Autodesk Inventor part; units mm, degrees
ref_plane "Начальная плоскость" through (0, 0, 0) normal (0, 0, 1) x (1, 0, 0)
ref_plane "Конечная плоскость" through (0, 0, 1) normal (0, 0, 1) x (1, 0, 0)
ref_plane "YZ Plane" through (0, 0, 0) normal (1, 0, 0) x (0, 1, 0)
ref_plane "Начальная плоскость" through (0, 0, 0) normal (0, 0, 1) x (1, 0, 0)
ref_plane "Конечная плоскость" through (0, 0, 1) normal (0, 0, 1) x (1, 0, 0)
sketch "Эскиз" plane through (0, 0, 0) normal (0, 0, 1) x (1, 0, 0)
  line L0 (-13, -7) -> (-13, 43)
  line L1 (-17, 43) -> (-13, 43)
  line L2 (-17, -7) -> (-17, 43)
  line L3 (-7, -17) -> (33, -17)
  line L4 (33, -13) -> (33, -17)
  line L5 (-7, -13) -> (33, -13)
  arc A0 (-13, -7) -> (-7, -13) centre (-7, -7) ccw
  arc A1 (-17, -7) -> (-7, -17) centre (-7, -7) ccw
  line L6 (-17, 0) -> (23, 0) construction
  line L7 (0, -17) -> (0, 33) construction
  line L8 (0, 0) -> (50, 0) construction
  point P0 (-13, -13)
  point P1 (-17, -17)
  dimension "d17" = 6
  dimension "d18" = 10
  dimension "d25" = 17
  dimension "d26" = 17
  dimension "d27" = 90
  dimension "d28" = 50
  dimension "d29" = 60
  dimension "d30" = 4
  dimension "d31" = 4
  dimension "d32" = 50
extrude "Базовый элемент" add sketch "Эскиз" along normal up to surface (1 mm away) from surface at 0
sketch "Sketch3" plane through (0, 0, 0) normal (0, 0, 1) x (1, 0, 0)
  line L0 (0, 0) -> (10, 0)
ref_plane "Work Plane10" through (0, 0, 0) normal (0, -1, 0) x (1, 0, 0)
sketch "Sketch4" plane through (0, 0, 0) normal (0, -1, 0) x (1, 0, 0)
  line L0 (-2, 0) -> (12, 0)
  line L1 (-2, 1) -> (12, 1)
  dimension "d24" = 1
equation "\"d17\" = R"
equation "\"d18\" = R + ParT"
equation "\"d25\" = ey"
equation "\"d26\" = ex"
equation "\"d30\" = ParT"
equation "\"d31\" = ParT"
equation "\"d32\" = d28"
equation "\"d11\" = G_L"
equation "\"b\" = 60"
equation "\"ParT\" = 4"
equation "\"R\" = 6"
equation "\"G_L\" = d24"
equation "\"G_OFFSET_START\" = 0"
equation "\"G_OFFSET_END\" = 0"
equation "\"d20\" = G_OFFSET_END + B_L"
equation "\"ex\" = 17"
equation "\"ey\" = ex"
equation "\"B_L\" = 1"
equation "\"a\" = 50"
properties part number "ДСТУ 2254-93 (Гнутий рівнобокий)" material "С245 ДСТУ 8539"
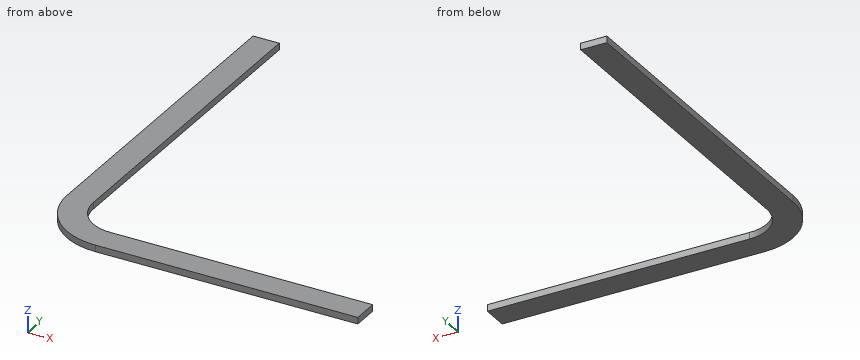
Source: CAD feature listing. Evaluate the final solid. Frame: model axes, mm. Give positions to 0.01 mm unless a question says otherwise; leave off trailing zeros. Order: outer loops, then holes, each group sorted by start corner. A loop starts at its lowest first (then second) coordinate and runs counter-clockwise, first axis right, second up.
(1) Section query A-A (z = 0.5). Return the cut outline in (x, y).
(2) Material intervals for line 1 along X through (y, z) = (37, 0.1); line 2 along X through (y, z) = (-12, 0.7), sorted ascending.
(3) Section query B-B (x = 3). Return the cut outline in (y, z), plus the area to 3 significant figures.
Outcome:
1. outline: (-17, -7) arc R10 ccw to (-7, -17) - (33, -17) - (33, -13) - (-7, -13) arc R6 cw to (-13, -7) - (-13, 43) - (-17, 43) - close
2. line 1: x = -17 to -13
2. line 2: x = -15.66 to -10.32
3. outline: (-17, 0) - (-13, 0) - (-13, 1) - (-17, 1) - close
3. area: 4.00 mm2
